Geometry check sheet. Reference: drawing and pictorial views, mm from the part's lowest x, y, z. A direction names the side the tool comes from. Round coordinates to 2 decimals unless told otherwise and drop trailing zeros. Order: outer loops, then holes, each group sorted by start corner. A loop starts at its lowest first (then second) coordinate and runs counter-clockwise, first axis right, second up.
Q1. Cross-section at A-A on z = 4. Record the cut outline in (x, y) (1 decimal).
Q2. Cross-section at B-B on y = 3.25. Record the cut outline in (x, z).
Q3. Cross-section at D-D on x = 6.5. Record the cut outline in (y, z), then the cut area to 3 significant figures.
Q4. Scan lines: probe 1 along X at (y, z) = (6, 14) (1 decimal); probe 2 along Y at (x, z) = (5.5, 12.25) (1 decimal); probe 3 along Y at (x, z) = (7, 11) (1 decimal). Record each from-to range of solid material in increasing order.
Q5. Depth check by flat-ended pin: P1, Ø1, axis at y = 2, z = 13, coming from the -X side; P2, Ø2, axis at x = 5.5, y = 6, coming from the +Z side; P3, Ø1.5, axis at x = 8, z = 8.5, coming from the -Y side (1 decimal); P4, Ø5, axis at x = 10, z = 9.5, coming from the +Y side. Enter the tip coordinate at first touch or a pass-through.
Q6. Mould release check, pull along X, two halves, no side actions. Record for the marked faces 3, 4, 5 and 6: +X half, -X half, draft (parallel to the pull), parting line (faces both ways), or undercut.
Q7. Cross-section at C-C on z = 15.5. Record the cut outline in (x, y) (1 decimal).
Q8. Set-up check for the marked faces 1 and 2: record each of +Z, -Z, +X, -X, +Y, -Y from which the full face is reachable in a straight line by a thin tool's end or side.
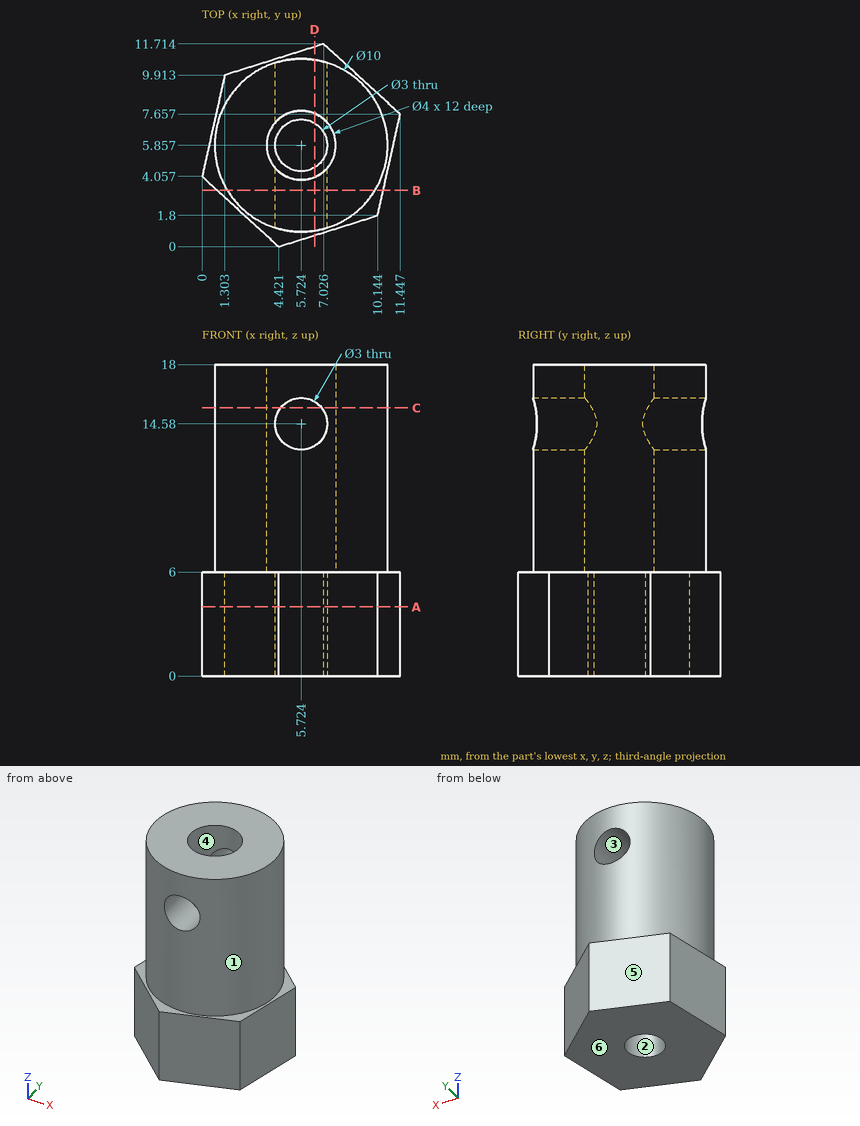
Results found:
1. outline: (0, 4.1) - (4.4, 0) - (10.1, 1.8) - (11.4, 7.7) - (7, 11.7) - (1.3, 9.9) - close; hole circle Ø3 at (5.7, 5.9)
2. outline: (0.88, 0) - (10.47, 0) - (10.47, 6) - (9.99, 6) - (9.99, 18) - (1.46, 18) - (1.46, 6) - (0.88, 6) - close; hole circle Ø3 at (5.72, 14.58)
3. outline: (0.65, 0) - (4.57, 0) - (4.57, 6) - (4.01, 6) - (4.01, 13.3) - (0.92, 13.3) - (0.92, 6) - (0.65, 6) - close; (0.92, 15.86) - (4.01, 15.86) - (4.01, 18) - (0.92, 18) - close; (7.14, 0) - (11.55, 0) - (11.55, 6) - (10.8, 6) - (10.8, 13.3) - (7.7, 13.3) - (7.7, 6) - (7.14, 6) - close; (7.7, 15.86) - (10.8, 15.86) - (10.8, 18) - (7.7, 18) - close
3. area: 108 mm2
4. probe 1: x = 0.7 to 3.7, 7.7 to 10.7
4. probe 2: y = 0.9 to 3.9, 7.8 to 10.9
4. probe 3: y = 1 to 4.3, 7.4 to 10.7
5. P1: stops at x = 2.02
5. P2: passes through
5. P3: stops at y = 1.1
5. P4: stops at y = 10.53
6. face 3: undercut
6. face 4: undercut
6. face 5: -X half
6. face 6: draft
7. outline: (4.5, 1) - (4.5, 4.2) arc R2 cw to (4.5, 7.5) - (4.5, 10.7) arc R5 ccw to start; (6.9, 1) arc R5 ccw to (6.9, 10.7) - (6.9, 7.5) arc R2 cw to (6.9, 4.2) - close
8. face 1: +Z
8. face 2: +Z, -Z
